```python
from build123d import *

# Parameters (mm, degrees)
SKETCH1_W           = 313
SKETCH1_H           = 342
BOSS_EXTRUDE1_DEPTH = 6.35
SKETCH3_W           = 22
SKETCH3_H           = 155.14040353
SKETCH3_R           = 2.5
BOSS_EXTRUDE2_DEPTH = 6.35
SKETCH2_R           = 2.5
CUT_EXTRUDE1_DEPTH  = 248.272263912
SKETCH4_R           = 3.5
CUT_EXTRUDE2_DEPTH  = 248.272263912


with BuildPart() as part:
    # Sketch1 → Boss-Extrude1 (new body)
    with BuildSketch(Plane(origin=(0, 0, 0), x_dir=(1, 0, 0), z_dir=(0, 1, 0))):
        Rectangle(SKETCH1_W, SKETCH1_H)
    extrude(amount=-BOSS_EXTRUDE1_DEPTH)

    # Sketch3 → Boss-Extrude2 (add)
    with BuildSketch(Plane(origin=(0, 0, 0), x_dir=(1, 0, 0), z_dir=(0, 1, 0))):
        with Locations((167.5, 9)):
            Rectangle(SKETCH3_W, SKETCH3_H)
        with Locations(Location((166.5, 9, 0), (0, 0, 270))):
            Circle(SKETCH3_R, mode=Mode.SUBTRACT)
        with Locations(Location((166.5, -41.8, 0), (0, 0, 270))):
            Circle(SKETCH3_R, mode=Mode.SUBTRACT)
        with Locations(Location((166.5, 59.8, 0), (0, 0, 90))):
            Circle(SKETCH3_R, mode=Mode.SUBTRACT)
    extrude(amount=-BOSS_EXTRUDE2_DEPTH)

    # Sketch2 → Cut-Extrude1 (cut, through all)
    with BuildSketch(Plane(origin=(0, 0, 0), x_dir=(1, 0, 0), z_dir=(0, 1, 0))):
        with Locations(Location((0, -123, 0), (0, 0, 270))):
            Circle(SKETCH2_R)
        with Locations(Location((-70, -123, 0), (0, 0, 270))):
            Circle(SKETCH2_R)
        with Locations(Location((70, -123, 0), (0, 0, 90))):
            Circle(SKETCH2_R)
        with Locations(Location((-70, 141, 0), (0, 0, 90))):
            Circle(SKETCH2_R)
        with Locations(Location((0, 141, 0), (0, 0, 90))):
            Circle(SKETCH2_R)
        with Locations(Location((70, 141, 0), (0, 0, 270))):
            Circle(SKETCH2_R)
    extrude(amount=-CUT_EXTRUDE1_DEPTH, mode=Mode.SUBTRACT)

    # Sketch4 → Cut-Extrude2 (cut, through all)
    with BuildSketch(Plane(origin=(0, 0, 0), x_dir=(1, 0, 0), z_dir=(0, 1, 0))):
        with Locations(Location((133.64, -142.84, 0), (0, 0, 270))):
            Circle(SKETCH4_R)
        with Locations(Location((108.24, -142.84, 0), (0, 0, 270))):
            Circle(SKETCH4_R)
    cut_extrude2 = extrude(amount=-CUT_EXTRUDE2_DEPTH, mode=Mode.SUBTRACT)

    # Mirror1: Cut-Extrude2 across plane
    add(cut_extrude2.mirror(Plane(origin=(0, 0, -9), x_dir=(1, 0, 0), z_dir=(0, 0, -1))), mode=Mode.SUBTRACT)


solid = part.part
```
Check sheet for the modelled part. Datum: model origin and axes. Units: mm. Give positions to 0.01 mm unless a question says otherwise; leave off trailing zeros. Write each loop counter-clockwise with the first axis right and the second up, starting at its lowest first coordinate (ties: lowest second). Pieces come first, ordered by that corner, then holes. Notation, with made-up numbers: (-7.5, -34) - (34.5, -34) arc R32 ccw to (34.5, 5) - close; hole circle Ø3 at (46.5, 29.5). An arc over 180 degrees is marked (long way). Answer as a JSON object with one key per item and string values. Group by question number.
1) Sectioned sample at B-B (z = -129.5). Record the cut outline in (x, y), then the cut area to 3 significant figures.
2) Depth check by flat-ended pin: P1, Ø4, axis at x = -70, z = 123, coming from the -Y side; P2, Ø1.9, axis at x = 170.5, y = -2.5, coming from the -Z side. Enter the tip coordinate at first touch or a pass-through.
3) Thickness scan on probe 1 along X at (y, z) = (-3.25, -141); probe 2 along X at (y, z) = (-2, 101); probe 3 along Z at (x, y) = (162, -2). Record the ranges inside material, lowest first. Write a range as from..to.
4) Sectioned sample at A-A (y = -5). Give the number of separate pieces and of enclosed holes in the cut face, then the cut area to 3 significant figures.
Geometry results:
{
 "1": {"outline": "(-156.5, -6.35) - (156.5, -6.35) - (156.5, 0) - (-156.5, 0) - close", "area": "1,990 mm^2"},
 "2": {"P1": "passes through", "P2": "stops at z = -86.57"},
 "3": {"probe 1": "x = -156.5..-72.5, -67.5..-2.5, 2.5..67.5, 72.5..156.5", "probe 2": "x = -156.5..156.5", "probe 3": "z = -86.57..68.57"},
 "4": {"separate pieces": "1", "enclosed holes": "13", "area": "110,000 mm^2"}
}
